```python
from build123d import *

# Parameters (mm, degrees)
SKETCH1_W                      = 127
SKETCH1_H                      = 406.4
BOSS_EXTRUDE1_DEPTH            = 1.5875
EDGE_FLANGE1_STRIP_W           = 9.525
EDGE_FLANGE1_STRIP_H           = 1.5875
EDGE_FLANGE1_STRIP_CUT_DEPTH   = 406.4
EDGE_FLANGE1_STRIP_2_W         = 9.525
EDGE_FLANGE1_STRIP_2_H         = 1.5875
EDGE_FLANGE1_STRIP_CUT_2_DEPTH = 406.4
EDGE_FLANGE1_DEPTH             = 406.4
EDGE_FLANGE1_BEND_DEPTH        = 406.4


# Sheet-metal steps are written as plain solids
with BuildPart() as part:
    # Sketch1 → Boss-Extrude1 (new body)
    with BuildSketch(Plane.XY):
        with Locations((63.5, 203.2)):
            Rectangle(SKETCH1_W, SKETCH1_H)
    extrude(amount=BOSS_EXTRUDE1_DEPTH)

    # Edge-Flange1 strip (across the edge) → Edge-Flange1 strip cut (cut)
    with BuildSketch(Plane(origin=(127, 0, 1.5875), x_dir=(-1, 0, 0), z_dir=(0, 1, 0))):
        with Locations((-1.5875, -0.79375)):
            Rectangle(EDGE_FLANGE1_STRIP_W, EDGE_FLANGE1_STRIP_H)
    extrude(amount=EDGE_FLANGE1_STRIP_CUT_DEPTH, mode=Mode.SUBTRACT)

    # Edge-Flange1 strip 2 (across the edge) → Edge-Flange1 strip cut 2 (cut)
    with BuildSketch(Plane(origin=(0, 406.4, 1.5875), x_dir=(1, 0, 0), z_dir=(0, -1, 0))):
        with Locations((-1.5875, -0.79375)):
            Rectangle(EDGE_FLANGE1_STRIP_2_W, EDGE_FLANGE1_STRIP_2_H)
    extrude(amount=EDGE_FLANGE1_STRIP_CUT_2_DEPTH, mode=Mode.SUBTRACT)

    # Edge-Flange1 section (across the edge) → Edge-Flange1 (add)
    with BuildSketch(Plane(origin=(127, 0, 1.5875), x_dir=(-1, 0, 0), z_dir=(0, 1, 0))):
        with BuildLine():
            Line((0, 1.5875), (0, 23.8125))
            Line((0, 23.8125), (1.5875, 23.8125))
            Line((1.5875, 23.8125), (1.5875, 1.5875))
            ThreePointArc((1.5875, 1.5875), (2.052467985, 0.464967985), (3.175, 0))
            Line((3.175, 0), (3.175, -1.5875))
            ThreePointArc((3.175, -1.5875), (0.92993597, -0.65756403), (0, 1.5875))
        make_face()
    extrude(amount=EDGE_FLANGE1_DEPTH)

    # Edge-Flange1 section 2 (across the edge) → Edge-Flange1 bend (add)
    with BuildSketch(Plane(origin=(0, 406.4, 1.5875), x_dir=(1, 0, 0), z_dir=(0, -1, 0))):
        with BuildLine():
            Line((0, 1.5875), (0, 23.8125))
            Line((0, 23.8125), (1.5875, 23.8125))
            Line((1.5875, 23.8125), (1.5875, 1.5875))
            ThreePointArc((1.5875, 1.5875), (2.052467985, 0.464967985), (3.175, 0))
            Line((3.175, 0), (3.175, -1.5875))
            ThreePointArc((3.175, -1.5875), (0.92993597, -0.65756403), (0, 1.5875))
        make_face()
    extrude(amount=EDGE_FLANGE1_BEND_DEPTH)


solid = part.part
```
Geometry: final body of the model. Coordinates: model frame, mm. A direction names the side the tool comes from. Coordinates: 2 decimals unless noted, no trailing zeros. Write each loop counter-clockwise with the first axis right and the second up, starting at its lowest first coordinate (ties: lowest second). Pieces come first, ordered by that corner, then holes. Notation, with made-up numbers: M 49,37 L 58,37 A23 ccw 58,47 Z; hole C 80.5,44 d10. An arc over 180 degrees is marked long. Use CSV: the item, a comma, the result in double quotes. Start each with the question number.
1. Mould query, pull axis X, two halves, no side actions, for faces 3 (the face through (64, 406.4, 1)), 4 (the face through (125.412, 200, 14)), 5 (the face through (0, 206, 14)). Classes: pulls with the +X half, pulls with the -X half, needs draft (parallel to the pull), parting line crosses it, or undercut.
2. Ray query, probe 1 along X at (y, z) = (18.5, 12.75); probe 2 along Z at (x, y) = (50.5, 78); probe 3 along X at (y, z) = (375, 2.5). Return the intervals inside material, ascending.
3. Cut plane A-A on z = 9. Return the cut outline in (x, y), plus the area to 3 significant figures.
4. First-contact query: P1, Ø2, axis at x = 91.5, z = 4.5, coming from the +Y side; P2, Ø2, axis at x = 74, y = 202.5, coming from the +Z side. Flat tips, straight axial feed; report the tip coordinate or a pass-through.
5. Reachability of faces 1 (the face through (1.588, 206, 14)), 2 (the face through (64, 0, 1)) from +Z, -Z, +X, -X, +Y, -Y: full face, straight path, thin tool, end or side. Return the list, or none.
6. Cut plane C-C on x = 14. Return the cut outline in (y, z), plus the area to 3 significant figures.
Entries:
1,face 3,"needs draft"
1,face 4,"undercut"
1,face 5,"pulls with the -X half"
2,probe 1,"0 to 1.59, 125.41 to 127"
2,probe 2,"0 to 1.59"
2,probe 3,"0.07 to 1.74, 125.26 to 126.93"
3,outline,"M 0,0 L 1.59,0 L 1.59,406.4 L 0,406.4 Z; M 125.41,0 L 127,0 L 127,406.4 L 125.41,406.4 Z"
3,area,"1,290 mm²"
4,P1,"through"
4,P2,"z = 1.59"
5,face 1,"+Z, +Y, -Y"
5,face 2,"+Z, -Z, +X, -X, -Y"
6,outline,"M 0,0 L 406.4,0 L 406.4,1.59 L 0,1.59 Z"
6,area,"645 mm²"
